CAD build for the part. Positions are in the model's coordinates, mm. Face numbers are marked on the shaded views. A direction names the side the tool comes from. Coordinates: 2 decimals unless noted, no trailing zeros. Order: outer loops, then holes, each group sorted by start corner. A loop starts at its lowest first (then second) coordinate and runs counter-clockwise, first axis right, second up. Notation, with made-up numbers: M 63,-12 L 108,-12 A23 cw 108,8 Z; hole C 54.25,66 d1. An arc over 180 degrees is marked long. Write item = value, one per line. Start each with the question number.
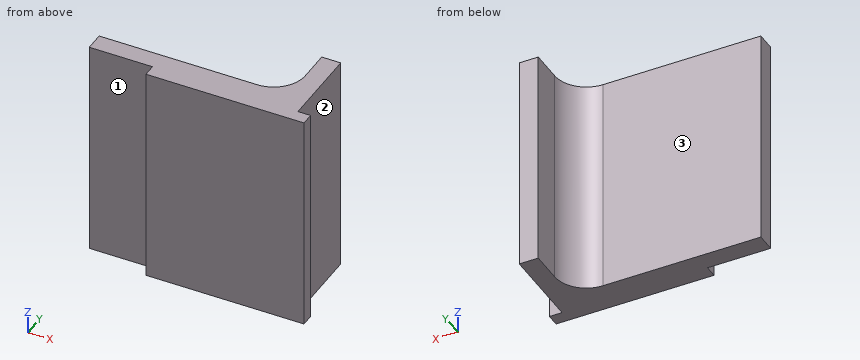
```python
from build123d import *

# Parameters (mm, degrees)
F1_DEPTH = 17.5
F2_R     = 5


with BuildPart() as f1:
    # F0 (on Top) → F1 (new body, symmetric)
    with BuildSketch(Plane.XY):
        Polygon((-6.7937952719, 3), (-36.7937952719, 3), (-36.7937952719, 0), (-26.7937952719, 0), (-26.7937952719, -2), (-3.7937952719, -2), (-1.7937952719, -2), (-1.7937952719, 0), (-3.7937952719, 0), (-3.7937952719, 13), (-6.7937952719, 13), align=None)
    extrude(amount=F1_DEPTH, both=True)

    # F2
    f2_edges = [f1.edges().sort_by_distance(p)[0] for p in [
        (-6.793795, 3, 0),
    ]]
    fillet(f2_edges, radius=F2_R)


solid = f1.part
```
1. 3-axis set-ups, long thin cutter, end or side, ignore diameter. For the marked faces 1, 2 and 3: which of +Z, -Z, +X, -X, +Y, -Y reach the whole face in a straight line?
2. Slice it at A-A (z = 2). Write the cut outline in (x, y), plus the area to 3 significant figures.
3. Slice it at C-C (x = -29). Write the cut outline in (y, z), plus the area to 3 significant figures.
4. Flat gauge pins, fed straight in: pin 1 (2 mm diameter, centred on y = -1.5, z = -5, fed in from -X); pin 2 (4 mm diameter, centred on y = 11.5, z = -4.5, fed in from -X); pin 3 (1.5 mm diameter, centred on y = 6.5, z = -6, fed in from +X). Where does each tip first touch, or does it go through?
5. Slice it at B-B (y = 0.5). Write the cut outline in (x, z).
6. Probe L1, parallel to Y at x = -28.5, z = -13.5; L2, parallel to Y at x = -12.5, z = -5; L3, parallel to X at y = 10, z = -15. List the from-to ranges inside material, lowest first.
Calculated:
q1.face_1 = +Z, -Z, -X, -Y
q1.face_2 = +Z, -Z, +X, +Y
q1.face_3 = +Z, -Z, -X, +Y
q2.outline = M -36.79,0 L -26.79,0 L -26.79,-2 L -1.79,-2 L -1.79,0 L -3.79,0 L -3.79,13 L -6.79,13 L -6.79,8 A5 cw -11.79,3 L -36.79,3 Z
q2.area = 184 mm²
q3.outline = M 0,-17.5 L 3,-17.5 L 3,17.5 L 0,17.5 Z
q3.area = 105 mm²
q4.pin_1 = -26.79
q4.pin_2 = -6.79
q4.pin_3 = -3.79
q5.outline = M -36.79,-17.5 L -3.79,-17.5 L -3.79,17.5 L -36.79,17.5 Z
q6.L1 = 0 to 3
q6.L2 = -2 to 3
q6.L3 = -6.79 to -3.79
